```python
from build123d import *

# Parameters (mm, degrees)
SKETCH1_R           = 1.25
SKETCH1_R_2         = 8.5
SKETCH1_R_3         = 1.5
SKETCH1_R_4         = 1.65
SKETCH1_R_5         = 2
BOSS_EXTRUDE1_DEPTH = 5
CHAMFER1_SIZE       = 0.5


with BuildPart() as part:
    # Sketch1 → Boss-Extrude1 (new body)
    with BuildSketch(Plane.XY):
        with BuildLine():
            Line((0, -10), (197.5, -10))
            ThreePointArc((197.5, -10), (202.096194078, -11.903805922), (204, -16.5))
            Line((204, -16.5), (204, -36.746197724))
            ThreePointArc((204, -36.746197724), (205.903805922, -41.342391801), (210.5, -43.246197724))
            Line((210.5, -43.246197724), (217.5, -43.246197724))
            ThreePointArc((217.5, -43.246197724), (222.096194078, -41.342391801), (224, -36.746197724))
            Line((224, -36.746197724), (224, -0.946197724))
            Line((224, -0.946197724), (206, -0.946197724))
            ThreePointArc((206, -0.946197724), (204.585786438, -0.360411286), (204, 1.053802276))
            Line((204, 1.053802276), (204, 15))
            Line((204, 15), (-9.5, 15))
            ThreePointArc((-9.5, 15), (-10.914213562, 15.585786438), (-11.5, 17))
            Line((-11.5, 17), (-11.5, 18))
            Line((-11.5, 18), (-46, 18))
            ThreePointArc((-46, 18), (-50.596194078, 16.096194078), (-52.5, 11.5))
            Line((-52.5, 11.5), (-52.5, -36.746197724))
            ThreePointArc((-52.5, -36.746197724), (-50.596194078, -41.342391801), (-46, -43.246197724))
            Line((-46, -43.246197724), (-13, -43.246197724))
            ThreePointArc((-13, -43.246197724), (-8.403805922, -41.342391801), (-6.5, -36.746197724))
            Line((-6.5, -36.746197724), (-6.5, -16.5))
            ThreePointArc((-6.5, -16.5), (-4.596194078, -11.903805922), (0, -10))
        make_face()
        Circle(SKETCH1_R, mode=Mode.SUBTRACT)
        with Locations((20, 0)):
            Circle(SKETCH1_R, mode=Mode.SUBTRACT)
        with Locations((40, 0)):
            Circle(SKETCH1_R, mode=Mode.SUBTRACT)
        with Locations((60, 0)):
            Circle(SKETCH1_R, mode=Mode.SUBTRACT)
        with Locations((80, 0)):
            Circle(SKETCH1_R, mode=Mode.SUBTRACT)
        with Locations((100, 0)):
            Circle(SKETCH1_R, mode=Mode.SUBTRACT)
        with Locations((120, 0)):
            Circle(SKETCH1_R, mode=Mode.SUBTRACT)
        with Locations((140, 0)):
            Circle(SKETCH1_R, mode=Mode.SUBTRACT)
        with Locations((160, 0)):
            Circle(SKETCH1_R, mode=Mode.SUBTRACT)
        with Locations((180, 0)):
            Circle(SKETCH1_R, mode=Mode.SUBTRACT)
        with Locations((-30, -20.746197724)):
            Circle(SKETCH1_R_2, mode=Mode.SUBTRACT)
        with Locations((-45.5, -5.246197724)):
            Circle(SKETCH1_R_3, mode=Mode.SUBTRACT)
        with Locations((-14.5, -5.246197724)):
            Circle(SKETCH1_R_3, mode=Mode.SUBTRACT)
        with Locations((-45.5, -36.246197724)):
            Circle(SKETCH1_R_3, mode=Mode.SUBTRACT)
        with Locations((-14.5, -36.246197724)):
            Circle(SKETCH1_R_3, mode=Mode.SUBTRACT)
        with Locations((200, 0)):
            Circle(SKETCH1_R, mode=Mode.SUBTRACT)
        with Locations((212, -20.746197724)):
            Circle(SKETCH1_R_4, mode=Mode.SUBTRACT)
        with Locations((214, -36.246197724)):
            Circle(SKETCH1_R_3, mode=Mode.SUBTRACT)
        with Locations((214, -5.246197724)):
            Circle(SKETCH1_R_3, mode=Mode.SUBTRACT)
        with Locations((-39.9, 6.9)):
            Circle(SKETCH1_R_5, mode=Mode.SUBTRACT)
        with BuildLine():
            Line((-20.9, 16), (-15.9, 16))
            ThreePointArc((-15.9, 16), (-14.485786438, 15.414213562), (-13.9, 14))
            Line((-13.9, 14), (-13.9, 12.12))
            ThreePointArc((-13.9, 12.12), (-14.485786438, 10.705786438), (-15.9, 10.12))
            Line((-15.9, 10.12), (-20.9, 10.12))
            ThreePointArc((-20.9, 10.12), (-22.314213562, 10.705786438), (-22.9, 12.12))
            Line((-22.9, 12.12), (-22.9, 14))
            ThreePointArc((-22.9, 14), (-22.314213562, 15.414213562), (-20.9, 16))
        make_face(mode=Mode.SUBTRACT)
        with BuildLine():
            Line((-26.9, 12.9), (-31.9, 12.9))
            ThreePointArc((-31.9, 12.9), (-33.314213562, 12.314213562), (-33.9, 10.9))
            Line((-33.9, 10.9), (-33.9, 2.9))
            ThreePointArc((-33.9, 2.9), (-33.314213562, 1.485786438), (-31.9, 0.9))
            Line((-31.9, 0.9), (-26.9, 0.9))
            ThreePointArc((-26.9, 0.9), (-25.485786438, 1.485786438), (-24.9, 2.9))
            Line((-24.9, 2.9), (-24.9, 10.9))
            ThreePointArc((-24.9, 10.9), (-25.485786438, 12.314213562), (-26.9, 12.9))
        make_face(mode=Mode.SUBTRACT)
    extrude(amount=BOSS_EXTRUDE1_DEPTH)

    # Chamfer1
    chamfer1_edges = [part.edges().sort_by_distance(p)[0] for p in [
        (-14.485786438, 15.414213562, 0),
        (-18.4, 16, 0),
        (-22.314213562, 15.414213562, 0),
        (-22.9, 13.06, 0),
        (-22.314213562, 10.705786438, 0),
        (-18.4, 10.12, 0),
        (-14.485786438, 10.705786438, 0),
        (-13.9, 13.06, 0),
        (-14.485786438, 15.414213562, 5),
        (-18.4, 16, 5),
        (-22.314213562, 15.414213562, 5),
        (-22.9, 13.06, 5),
        (-22.314213562, 10.705786438, 5),
        (-18.4, 10.12, 5),
        (-14.485786438, 10.705786438, 5),
        (-13.9, 13.06, 5),
        (205.903805922, -41.342391801, 5),
        (-25.485786438, 12.314213562, 0),
        (-29.4, 12.9, 0),
        (-33.314213562, 12.314213562, 0),
        (-33.9, 6.9, 0),
        (-33.314213562, 1.485786438, 0),
        (-29.4, 0.9, 0),
        (-25.485786438, 1.485786438, 0),
        (-24.9, 6.9, 0),
        (-25.485786438, 12.314213562, 5),
        (-29.4, 12.9, 5),
        (-33.314213562, 12.314213562, 5),
        (-33.9, 6.9, 5),
        (-33.314213562, 1.485786438, 5),
        (-29.4, 0.9, 5),
        (-25.485786438, 1.485786438, 5),
        (-24.9, 6.9, 5),
        (214, -43.246197724, 5),
        (-41.9, 6.9, 0),
        (-41.9, 6.9, 5),
        (98.75, -10, 0),
        (-4.596194078, -11.903805922, 0),
        (222.096194078, -41.342391801, 5),
        (-6.5, -26.623098862, 0),
        (-8.403805922, -41.342391801, 0),
        (-29.5, -43.246197724, 0),
        (-50.596194078, -41.342391801, 0),
        (-52.5, -12.623098862, 0),
        (-50.596194078, 16.096194078, 0),
        (-28.75, 18, 0),
        (-11.5, 17.5, 0),
        (-10.914213562, 15.585786438, 0),
        (97.25, 15, 0),
        (224, -18.846197724, 5),
        (204, 8.026901138, 0),
        (204.585786438, -0.360411286, 0),
        (215, -0.946197724, 0),
        (224, -18.846197724, 0),
        (222.096194078, -41.342391801, 0),
        (214, -43.246197724, 0),
        (205.903805922, -41.342391801, 0),
        (204, -26.623098862, 0),
        (202.096194078, -11.903805922, 0),
        (215, -0.946197724, 5),
        (204.585786438, -0.360411286, 5),
        (204, 8.026901138, 5),
        (97.25, 15, 5),
        (-10.914213562, 15.585786438, 5),
        (-11.5, 17.5, 5),
        (202.096194078, -11.903805922, 5),
        (-28.75, 18, 5),
        (-50.596194078, 16.096194078, 5),
        (-52.5, -12.623098862, 5),
        (-50.596194078, -41.342391801, 5),
        (-29.5, -43.246197724, 5),
        (-8.403805922, -41.342391801, 5),
        (-6.5, -26.623098862, 5),
        (-4.596194078, -11.903805922, 5),
        (98.75, -10, 5),
        (204, -26.623098862, 5),
    ]]
    chamfer(chamfer1_edges, length=CHAMFER1_SIZE)


solid = part.part
```
The listing builds one solid part. Answer for the finished solid, in the listing's coordinates (mm). A direction names the side the tool comes from. Round coordinates to 2 decimals unless told otherwise and drop trailing zeros. Write each loop counter-clockwise with the first axis right and the second up, starting at its lowest first coordinate (ties: lowest second). Pieces come first, ordered by that corner, then holes. Notation, with made-up numbers: (-24.75, -1) -> (15.25, -1) arc R33 cw to (15.25, 29) -> close; hole circle Ø9 at (29.5, 68.25). An arc over 180 degrees is marked (long way). Answer as a JSON object with one key per item and string values. Group by question number.
Q1. Section B-B (x = 189) is taken. Write down the section's boundary in (y, z).
Q2. Each of these flat-tipped pins is pushed along its axis until it touches: pin 1 Ø1 at (x, z) = (81.5, 0.5) entering from +Y; pin 2 Ø1 at (y, z) = (2.5, 0.5) entering from +X; pin 3 Ø2.5 at (x, y) = (-45.5, -5.25) entering from +Z; pin 4 Ø0.8 at (y, z) = (17.5, 2.5) entering from +X. Where does it stop, or does it pass through?
Q3. Straight lines are drawn through the part: line 1 along X through (y, z) = (-36, 1.9); line 2 along X through (y, z) = (-20.5, 1.5); line 3 along Y through (x, z) = (214, 2.1). For each, find the intervals that lie inside material, in ascending order.
Q4. Section A-A (y = -32) is taken. Write down the section's boundary in (x, z), plus the area to 3 significant figures.
Q5. Which of the six approach directions +Z, -Z, +X, -X, +Y, -Y give full straight-line access (tool end or side, diameter ignored) to faces 4 (the face through (205.85, -41.29, 2.47)), 5 (the face through (221.79, -41.132, 0.135)), 6 (the face through (206.11, -41.04, 0.14)), 7 (the face through (206.11, -41.04, 4.86)), 8 (the face through (-50.29, 15.89, 4.86))?
Q6. Section C-C (z = 3) is taken. Count the separate pieces of the cut face and the enclosed holes in it, plus the area to 3 significant figures.
Q7. Determine the mould class of faces 1 (the face through (-4.75, -11.86, 4.64)), 2 (the face through (-21.893, -18.193, 2.465)), 3 (the face through (-50.545, 16.146, 2.472)) for opening direction Y: pulls with the +Y half, pulls with the -Y half, needs draft (parallel to the pull), parting line crosses it, or undercut.
Check values:
{
 "1": {"outline": "(-10, 0.5) -> (-9.5, 0) -> (14.5, 0) -> (15, 0.5) -> (15, 4.5) -> (14.5, 5) -> (-9.5, 5) -> (-10, 4.5) -> close"},
 "2": {"pin 1": "y = 15", "pin 2": "x = 204", "pin 3": "through", "pin 4": "x = -11.5"},
 "3": {"line 1": "-52.5 to -46.98, -44.02 to -15.98, -13.02 to -6.5, 204 to 212.52, 215.48 to 224", "line 2": "-52.5 to -38.5, -21.5 to -6.5, 204 to 210.37, 213.63 to 224", "line 3": "-43.25 to -37.75, -34.75 to -6.75, -3.75 to -0.95"},
 "4": {"outline": "(-52.5, 0.5) -> (-52, 0) -> (-7, 0) -> (-6.5, 0.5) -> (-6.5, 4.5) -> (-7, 5) -> (-52, 5) -> (-52.5, 4.5) -> close; (204, 0.5) -> (204.5, 0) -> (223.5, 0) -> (224, 0.5) -> (224, 4.5) -> (223.5, 5) -> (204.5, 5) -> (204, 4.5) -> close", "area": "329 mm^2"},
 "5": {"face 4": "+Z, -Z, -Y", "face 5": "-Z, +X, -Y", "face 6": "-Z, -Y", "face 7": "+Z, -Y", "face 8": "+Z, -X, +Y"},
 "6": {"separate pieces": "1", "enclosed holes": "22", "area": "8,390 mm^2"},
 "7": {"face 1": "pulls with the -Y half", "face 2": "undercut", "face 3": "pulls with the +Y half"}
}
